```python
from build123d import *

# Parameters (mm, degrees)
ESQUISSE1_R             = 28
BOSS_EXTRU_1_DEPTH      = 20
CHANFREIN1_SIZE         = 0.2
CHANFREIN1_SIZE2        = 0.266833281
ESQUISSE3_R             = 2
BOSS_EXTRU_2_DEPTH      = 3.5
ESQUISSE4_R             = 1.5
ENL_V_MAT_EXTRU_1_DEPTH = 5
ESQUISSE5_R             = 1.5
ENL_V_MAT_EXTRU_2_DEPTH = 10


with BuildPart() as part:
    # Esquisse1 → Boss.-Extru.1 (new body)
    with BuildSketch(Plane(origin=(0, 0, 0), x_dir=(1, 0, 0), z_dir=(0, 1, 0))):
        with Locations(Location((0, 0, 0), (0, 0, 270))):
            Circle(ESQUISSE1_R)
    extrude(amount=BOSS_EXTRU_1_DEPTH)

    # Esquisse2 → Enlèvement de matière-Révolution1 (revolve, cut)
    with BuildSketch(Plane(origin=(0, 0, 0), x_dir=(0, 0, -1), z_dir=(1, 0, 0))):
        Polygon((-28, 20), (-28, 17), (-15, 20), align=None)
    revolve(axis=Axis((0, 20, 0), (0, -1, 0)), mode=Mode.SUBTRACT)

    # Chanfrein1
    chanfrein1_edges = [part.edges().sort_by_distance(p)[0] for p in [
        (0, 17, -28),
    ]]
    chanfrein1_side = [part.faces().sort_by_distance(p)[0] for p in [
        (0, 8.5, -28),
    ]]
    chamfer(chanfrein1_edges, length=CHANFREIN1_SIZE, length2=CHANFREIN1_SIZE2, reference=chanfrein1_side[0])

    # Esquisse3 → Boss.-Extru.2 (add)
    with BuildSketch(Plane(origin=(0, 20, 0), x_dir=(1, 0, 0), z_dir=(0, 1, 0))):
        with Locations(Location((0, 0, 0), (0, 0, 270))):
            Circle(ESQUISSE3_R)
    extrude(amount=BOSS_EXTRU_2_DEPTH)

    # Esquisse4 → Enlèv. mat.-Extru.1 (cut)
    with BuildSketch(Plane(origin=(0, 20, 0), x_dir=(1, 0, 0), z_dir=(0, 1, 0))):
        with Locations(Location((0, 6, 0), (0, 0, 270))):
            Circle(ESQUISSE4_R)
        with Locations(Location((6, 0, 0), (0, 0, 270))):
            Circle(ESQUISSE4_R)
        with Locations(Location((0, -6, 0), (0, 0, 270))):
            Circle(ESQUISSE4_R)
        with Locations(Location((-6, 0, 0), (0, 0, 270))):
            Circle(ESQUISSE4_R)
    extrude(amount=-ENL_V_MAT_EXTRU_1_DEPTH, mode=Mode.SUBTRACT)

    # Esquisse5 → Enlèv. mat.-Extru.2 (cut)
    with BuildSketch(Plane(origin=(0, 20, 0), x_dir=(1, 0, 0), z_dir=(0, 1, 0))):
        with Locations(Location((-5.656854249, 5.656854249, 0), (0, 0, 270))):
            Circle(ESQUISSE5_R)
        with Locations(Location((5.656854249, 5.656854249, 0), (0, 0, 270))):
            Circle(ESQUISSE5_R)
        with Locations(Location((5.656854249, -5.656854249, 0), (0, 0, 270))):
            Circle(ESQUISSE5_R)
        with Locations(Location((-5.656854249, -5.656854249, 0), (0, 0, 270))):
            Circle(ESQUISSE5_R)
    extrude(amount=-ENL_V_MAT_EXTRU_2_DEPTH, mode=Mode.SUBTRACT)


solid = part.part
```
The listing builds one solid part. Answer for the finished solid, in the listing's coordinates (mm). A direction names the side the tool comes from. Give positions to 0.01 mm unless a question says otherwise; leave off trailing zeros. Order: outer loops, then holes, each group sorted by start corner. A loop starts at its lowest first (then second) coordinate and runs counter-clockwise, first axis right, second up.
Item 1: The part is cut by section B-B, the plane y = 12. Give the vertices of the cut face in (x, z), and give its area (3 significant figures).
From the geometry:
outline: circle Ø56 at (0, 0); hole circle Ø3 at (-5.66, -5.66); hole circle Ø3 at (-5.66, 5.66); hole circle Ø3 at (5.66, -5.66); hole circle Ø3 at (5.66, 5.66)
area: 2,430 mm2
Item 2: For a pull along Z with two mould halves and no side action, classify faces 3 (the face through (5.982, 19.857, 14.428)), 4 (the face through (4.3, 15.1, 6.3)), 5 (the face through (0, 0, 0)) as pulls with the +Z half, pulls with the -Z half, needs draft (parallel to the pull), parting line crosses it, or undercut.
From the geometry:
face 3: parting line crosses it
face 4: undercut
face 5: needs draft
Item 3: The part is cut by section A-A, the plane y = 22.25. Give the vertices of the cut face in (x, z).
From the geometry:
outline: circle Ø4 at (0, 0)
Item 4: The part is cut by section C-C, the plane y = 4.5. Give the vertices of the cut face in (x, z), and give its area (3 significant figures).
From the geometry:
outline: circle Ø56 at (0, 0)
area: 2,460 mm2
Item 5: Find the intervals of material crossed by probe 1 along X at (y, z) = (16.2, -6); probe 2 along Y at (x, z) = (5, -12); probe 3 along Y at (x, z) = (-21.5, 13.5), in increasing order.
From the geometry:
probe 1: x = -27.35 to -7.12, -4.2 to -1.5, 1.5 to 4.2, 7.12 to 27.35
probe 2: y = 0 to 20
probe 3: y = 0 to 17.6
Item 6: Given pin 1 Ø12 at (x, y) = (19, 5) entering from -Z; pin 2 Ø0.9 at (x, z) = (-5, -6) entering from +Y; pin 3 Ø2 at (y, z) = (17, 3) entering from -X, each flat-ended and moving along its own axis, determine where each tip first touches the part or whether it passes through.
From the geometry:
pin 1: stops at z = -24.8
pin 2: stops at y = 10
pin 3: stops at x = -27.93
Item 7: Which of the six approach directions +Z, -Z, +X, -X, +Y, -Y give full straight-line access (tool end or side, diameter ignored) to faces 1 (the face through (23.61, 8.28, 15.05)), 2 (the face through (0.07, 17.54, 4.5))?
From the geometry:
face 1: +Y, -Y
face 2: +Y
